Build history of the part. All positions in model axes, mm. Face numbers are marked on the shaded views. A direction names the side the tool comes from. Give positions to 0.01 mm unless a question says otherwise; leave off trailing zeros. Order: outer loops, then holes, each group sorted by start corner. A loop starts at its lowest first (then second) coordinate and runs counter-clockwise, first axis right, second up. Notation, with made-up numbers: (75, -16.75) - (132, -16.75) arc R25 cw to (132, -4.75) - close; hole circle Ø11 at (-20.75, 85.25). An arc over 180 degrees is marked (long way). Write each question's results on one line, items separated by ' | '. Start each with the question number.
from build123d import *

# Parameters (mm, degrees)
F2_W      = 60
F2_H      = 40
F3_DEPTH  = 140
F3_TAPER  = 3
F4_W      = 30
F4_H      = 20
F5_DEPTH  = 150
F6_R      = 4.5
F6_R_2    = 2
F7_DEPTH  = 150
F8_W      = 30
F8_H      = 25
F9_DEPTH  = 150
F10_W     = 93.8083151965
F10_H     = 20
F11_DEPTH = 70.001


with BuildPart() as f1:
    # F0 (on Right) → F1 (revolve)
    with BuildSketch(Plane.YZ):
        Polygon((-65, 0), (-52, 0), (-50.5, 50), (0, 50), (0, 70), (-65, 70), align=None)
    revolve(axis=Axis((0, 0, 53.9928800981), (0, 0, 1)))

    # F2 (on face) → F3 (join)
    with BuildSketch(Plane.XY.offset(70)):
        Rectangle(F2_W, F2_H)
    extrude(amount=F3_DEPTH, taper=F3_TAPER)

    # F4 (on Right) → F5 (cut, symmetric)
    with BuildSketch(Plane.YZ):
        with Locations((-25, 150)):
            Rectangle(F4_W, F4_H)
        with Locations((25, 150)):
            Rectangle(F4_W, F4_H)
    extrude(amount=F5_DEPTH, both=True, mode=Mode.SUBTRACT)

    # F6 (on face) → F7 (cut, symmetric)
    with BuildSketch(Plane.XZ.offset(10)):
        with Locations((0, 150)):
            Circle(F6_R)
        with Locations((0, 200)):
            Circle(F6_R_2)
    extrude(amount=F7_DEPTH, both=True, mode=Mode.SUBTRACT)

    # F8 (on Right) → F9 (cut, symmetric)
    with BuildSketch(Plane.YZ):
        with Locations((-19, 197.5)):
            Rectangle(F8_W, F8_H)
        with Locations((19, 197.5)):
            Rectangle(F8_W, F8_H)
    extrude(amount=F9_DEPTH, both=True, mode=Mode.SUBTRACT)

    # F10 (on face) → F11 (cut, through all)
    with BuildSketch(Plane.XY.offset(70)):
        with Locations((0, 55)):
            Rectangle(F10_W, F10_H)
    extrude(amount=-F11_DEPTH, mode=Mode.SUBTRACT)


solid = f1.part
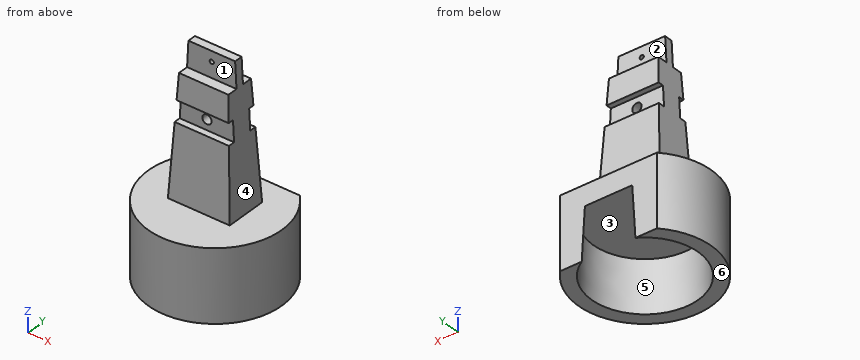
Item 1: Two-plate mould, pull along X, no slides. Class the marked faces 4, 5 and 6: +X half, -X half, draft (parallel to the pull), parting line (faces both ways), or undercut.
Item 2: Cut at B-B, the plane z = 63. List the corners of the cut face in (x, y), then the cut area to 3 significant figures.
Item 3: Probe line 1 along Z through (x, y) = (0, -2); line 2 along Z through (x, y) = (-55, -25.5); line 3 along Z through (x, y) = (19, 7). List the from-to ranges inside material, lowest first. Write a range as from..to.
Item 4: Which spindle directions (+Z, -Z, +X, -X, +Y, -Y) get a long thin tool onto all of the face, cutting with end or side? Do the marked faces 1, 2 and 3. Say none if no direction does.
Item 5: Cut at A-A, the plane y = 0. List the corners of the cut face in (x, z).
Item 6: Flat gauge pins, fed straight in: pin 1 Ø22 at (x, z) = (2.5, 145.5) entering from -Y; pin 2 Ø2 at (y, z) = (-25, 62) entering from +X; pin 3 Ø12 at (x, y) = (-21, 14) entering from -Z. Where does each tip first touch, or does it go through?
Item 7: Cut at C-C, the plane y = -55.5. List the corners of the cut face in (x, z), then the cut area to 3 significant figures.
Item 8: Cut at D-D, the plane z = 104.5. List the corners of the cut face in (x, y), then the cut area to 3 significant figures.
Values found:
1) face 4: +X half | face 5: undercut | face 6: draft
2) outline: (-46.9, 45) arc R65 ccw (long way) to (46.9, 45) - close | area: 12,000 mm2
3) line 1: z = 50..145.5, 154.5..198, 202..210 | line 2: z = 0..70 | line 3: z = 50..185
4) face 1: +Z, +X, -X, -Y | face 2: +Z, +X, -X, +Y | face 3: -Z
5) outline: (-65, 0) - (-52, 0) - (-50.5, 50) - (50.5, 50) - (52, 0) - (65, 0) - (65, 70) - (30, 70) - (22.66, 210) - (-22.66, 210) - (-30, 70) - (-65, 70) - close; hole circle Ø9 at (0, 150); hole circle Ø4 at (0, 200)
6) pin 1: stops at y = -16.62 | pin 2: stops at x = 60.41 | pin 3: stops at z = 50
7) outline: (-33.83, 0) - (33.83, 0) - (33.83, 70) - (-33.83, 70) - close | area: 4,740 mm2
8) outline: (-28.19, -18.19) - (28.19, -18.19) - (28.19, 18.19) - (-28.19, 18.19) - close | area: 2,050 mm2
